Source: CAD feature listing. Evaluate the final solid. Frame: model axes, mm. Face numbers are marked on the shaded views. A direction names the side the tool comes from. Coordinates: 2 decimals unless noted, no trailing zeros. Loops run counter-clockwise (first coordinate to the right, second up) from the corner with the lowest first, then second, coordinate; pieces in that order, holes last.
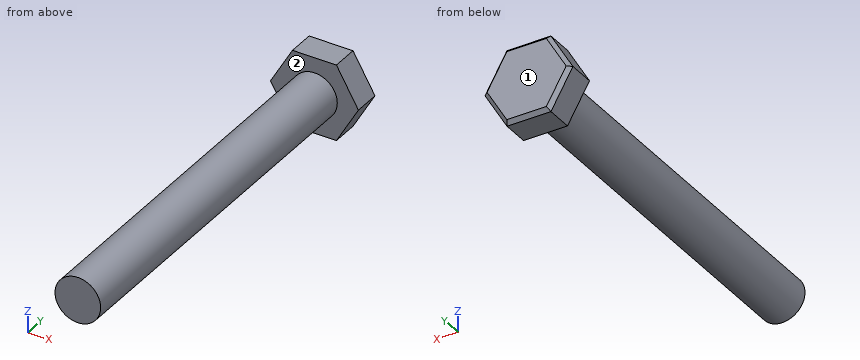
from build123d import *

# Parameters (mm, degrees)
F1_DEPTH = 4
F2_R     = 3
F3_DEPTH = 50
F4_SIZE  = 0.5


with BuildPart() as f1:
    # F0 (on Front) → F1 (new body)
    with BuildSketch(Plane.XZ):
        Polygon((2.886751, 5), (-2.886751, 5), (-5.773503, 0), (-2.886751, -5), (2.886751, -5), (5.773503, 0), align=None)
    extrude(amount=-F1_DEPTH)

    # F2 (on face) → F3 (join)
    with BuildSketch(Plane.XZ):
        Circle(F2_R)
    extrude(amount=F3_DEPTH)

    # F4
    f4_edges = [f1.edges().sort_by_distance(p)[0] for p in [
        (4.330127, 4, 2.5),
        (0, 4, 5),
        (-4.330127, 4, 2.5),
        (-4.330127, 4, -2.5),
        (0, 4, -5),
        (4.330127, 4, -2.5),
    ]]
    chamfer(f4_edges, length=F4_SIZE)


solid = f1.part
Q1. Section B-B, the plane y = -45. Return the cut outline in (x, z).
Q2. Access query for the marked faces 1 and 2. Directions: +Z, -Z, +X, -X, +Y, -Y. A direction counts if a zero-diameter tool reaches every point of the face in a straight line with its end or side. Return the directions, or none.
Q3. Section C-C, the plane z = -3.5. Return the cut outline in (x, y), plus the area to 3 significant figures.
Q4. Section A-A, the plane x = 0. Return the cut outline in (y, z), plus the area to 3 significant figures.
Q5. Section D-D, the plane x = -3.75. Return the cut outline in (y, z).
Q6. Line query: line 1 along X through (y, z) = (-36, 1.5); line 2 along Y through (x, z) = (3, -3.75); line 3 along Z through (x, y) = (2, -16.5). Output: solid intervals per line, ascending.
Q7. Contact query for flat-ended pins moving along their axis: pin 1 Ø6 at (x, y) = (-1.5, -38) entering from +Z; pin 2 Ø1.5 at (x, y) = (-4, -9) entering from -Z; pin 3 Ø4 at (y, z) = (-21, -1.5) entering from -X; pin 4 Ø3 at (y, z) = (-15, 2.5) entering from +X. Output: stop coordinate, or through.
Derived:
1. outline: circle Ø6 at (0, 0)
2. face 1: +Z, -Z, +X, -X, +Y
2. face 2: -Y
3. outline: (-3.75, 0) - (3.75, 0) - (3.75, 3.5) - (3.18, 4) - (-3.18, 4) - (-3.75, 3.5) - close
3. area: 29.7 mm2
4. outline: (-50, -3) - (0, -3) - (0, -5) - (3.5, -5) - (4, -4.5) - (4, 4.5) - (3.5, 5) - (0, 5) - (0, 3) - (-50, 3) - close
4. area: 340 mm2
5. outline: (0, -3.5) - (3.5, -3.5) - (4, -2.5) - (4, 2.5) - (3.5, 3.5) - (0, 3.5) - close
6. line 1: x = -2.6 to 2.6
6. line 2: y = 0 to 4
6. line 3: z = -2.24 to 2.24
7. pin 1: stops at z = 3
7. pin 2: passes through
7. pin 3: stops at x = -3
7. pin 4: stops at x = 2.83
